Can you work these out from the model? Positions are in its coordinate system, mm. Face numbers are marked on the shaded views. Round coordinates to 2 decimals unless told otherwise and drop trailing zeros. Loops run counter-clockwise (first coordinate to the right, second up) from the corner with the lowest first, then second, coordinate; pieces in that order, holes last. Notation, with made-up numbers: (69.25, -27) -> (119.25, -27) arc R27 ccw to (119.25, -5) -> close; hole circle Ø4 at (-18.75, 78). An arc over 180 degrees is marked (long way). Write each question's results on one line, items separated by ' | '.
from build123d import *

# Parameters (mm, degrees)
SKETCH5_W           = 58.42
SKETCH5_H           = 78.74
BOSS_EXTRUDE1_DEPTH = 1.5875
SKETCH6_R           = 0.381
BOSS_EXTRUDE2_DEPTH = 8.636
SKETCH7_W           = 2.54
SKETCH7_H           = 25.4
BOSS_EXTRUDE3_DEPTH = 8.382
SKETCH8_W           = 1.524
SKETCH8_H           = 0.762
SKETCH8_W_2         = 0.762
SKETCH8_H_2         = 1.524
BOSS_EXTRUDE4_DEPTH = 0.508


with BuildPart() as part:
    # Sketch5 → Boss-Extrude1 (new body)
    with BuildSketch(Plane(origin=(0, 0, 0), x_dir=(1, 0, 0), z_dir=(0, 1, 0))):
        with Locations((0, 13.97)):
            Rectangle(SKETCH5_W, SKETCH5_H)
    extrude(amount=BOSS_EXTRUDE1_DEPTH)

    # Sketch6 → Boss-Extrude2 (add)
    with BuildSketch(Plane(origin=(0, 1.5875, 0), x_dir=(1, 0, 0), z_dir=(0, 1, 0))):
        with Locations((-22.86, -21.59)):
            Circle(SKETCH6_R)
        with Locations((22.86, -21.59)):
            Circle(SKETCH6_R)
        with Locations((-22.86, -19.05)):
            Circle(SKETCH6_R)
        with Locations((22.86, -19.05)):
            Circle(SKETCH6_R)
        with Locations((-22.86, -16.51)):
            Circle(SKETCH6_R)
        with Locations((22.86, -16.51)):
            Circle(SKETCH6_R)
        with Locations((-22.86, -11.43)):
            Circle(SKETCH6_R)
        with Locations((22.86, -11.43)):
            Circle(SKETCH6_R)
        with Locations((-22.86, -8.89)):
            Circle(SKETCH6_R)
        with Locations((22.86, -8.89)):
            Circle(SKETCH6_R)
        with Locations((-22.86, -6.35)):
            Circle(SKETCH6_R)
        with Locations((22.86, -6.35)):
            Circle(SKETCH6_R)
        with Locations((-22.86, -3.81)):
            Circle(SKETCH6_R)
        with Locations((22.86, -3.81)):
            Circle(SKETCH6_R)
        with Locations((-22.86, -1.27)):
            Circle(SKETCH6_R)
        with Locations((22.86, -1.27)):
            Circle(SKETCH6_R)
        with Locations((-22.86, 1.27)):
            Circle(SKETCH6_R)
        with Locations((22.86, 1.27)):
            Circle(SKETCH6_R)
        with Locations((-22.86, 3.81)):
            Circle(SKETCH6_R)
        with Locations((22.86, 3.81)):
            Circle(SKETCH6_R)
        with Locations((-22.86, 6.35)):
            Circle(SKETCH6_R)
        with Locations((22.86, 6.35)):
            Circle(SKETCH6_R)
        with Locations((-22.86, 8.89)):
            Circle(SKETCH6_R)
        with Locations((22.86, 8.89)):
            Circle(SKETCH6_R)
        with Locations((-22.86, 11.43)):
            Circle(SKETCH6_R)
        with Locations((22.86, 11.43)):
            Circle(SKETCH6_R)
    extrude(amount=BOSS_EXTRUDE2_DEPTH)

    # Sketch7 → Boss-Extrude3 (add)
    with BuildSketch(Plane.XZ):
        with Locations((-22.86, 0)):
            Rectangle(SKETCH7_W, SKETCH7_H)
        with Locations((22.86, 0)):
            Rectangle(SKETCH7_W, SKETCH7_H)
    extrude(amount=BOSS_EXTRUDE3_DEPTH)

    # Sketch8 → Boss-Extrude4 (add)
    with BuildSketch(Plane(origin=(0, 1.5875, 0), x_dir=(1, 0, 0), z_dir=(0, 1, 0))):
        with Locations((13.97, -22.86)):
            Rectangle(SKETCH8_W, SKETCH8_H)
        with Locations((8.89, -20.32)):
            Rectangle(SKETCH8_W_2, SKETCH8_H_2)
        with Locations((-13.97, -22.86)):
            Rectangle(SKETCH8_W, SKETCH8_H)
    extrude(amount=BOSS_EXTRUDE4_DEPTH)


solid = part.part
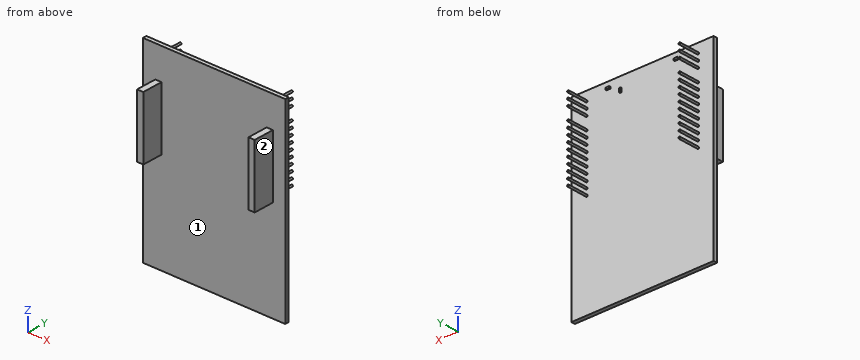
1. If we section it at D-D (x = -9): List the corners of the cut face in (y, z) for me.
Final values:
outline: (0, -53.34) -> (1.59, -53.34) -> (1.59, 25.4) -> (0, 25.4) -> close
2. Please list where these lines run through material, in increasing order: line 1 (X direction, y = -1, z = 5.5); line 2 (Y direction, x = -0.5, z = -24). Write a range as from..to.
Final values:
line 1: -24.13..-21.59, 21.59..24.13 | line 2: 0..1.59
3. If we section it at A-A (y = 3): State how many separate pieces and enclosed holes the cut face has, then the cut area to 3 significant figures.
Final values:
separate pieces: 26 | enclosed holes: 0 | area: 11.9 mm2
4. If we section it at C-C (z = -37): List the corners of the cut face in (x, y) for me, then the cut area to 3 significant figures.
Final values:
outline: (-29.21, 0) -> (29.21, 0) -> (29.21, 1.59) -> (-29.21, 1.59) -> close | area: 92.7 mm2
5. We'd pull the mould along X, two halves only. Please class the marked faces 1 and 2: pulls with the +X half, pulls with the -X half, needs draft (parallel to the pull), parting line crosses it, or undercut.
Final values:
face 1: undercut | face 2: pulls with the +X half
6. Will these pins go through, and if not, where does the flat tip stop? pin 1 (3 mm diameter, centred on x = -7, z = -25.5, fed in from -Y); pin 2 (1.3 mm diameter, centred on x = -23, y = -5, fed in from +Z); pin 3 (4 mm diameter, centred on y = -5, z = 2, fed in from -X); pin 4 (4 mm diameter, centred on x = -8.5, y = 5.5, fed in from +Z).
Final values:
pin 1: y = 0 | pin 2: z = 12.7 | pin 3: x = -24.13 | pin 4: through
7. If we section it at B-B (y = -3): List the corners of the cut face in (x, z) for me, then the cut area to 3 significant figures.
Final values:
outline: (-24.13, -12.7) -> (-21.59, -12.7) -> (-21.59, 12.7) -> (-24.13, 12.7) -> close; (21.59, -12.7) -> (24.13, -12.7) -> (24.13, 12.7) -> (21.59, 12.7) -> close | area: 129 mm2
